```python
from build123d import *

# Parameters (mm, degrees)
SKETCH1_R           = 1
BOSS_EXTRUDE1_DEPTH = 12
SKETCH2_R           = 3.3
CUT_EXTRUDE1_DEPTH  = 4.5
FILLET1_R           = 1
FILLET2_R           = 1


with BuildPart() as part:
    # Sketch1 → Boss-Extrude1 (new body)
    with BuildSketch(Plane.XY):
        with BuildLine():
            Line((-5.308637939, 12.706986515), (-5.308637939, 23.252630458))
            ThreePointArc((-5.308637939, 23.252630458), (-6.101385458, 28.176893504), (-1.247793812, 27.02821456))
            Line((-1.247793812, 27.02821456), (5.613218796, 27.02821456))
            Line((5.613218796, 27.02821456), (12.714242382, 53.529595368))
            ThreePointArc((12.714242382, 53.529595368), (11.748807445, 55.614439687), (11.81766691, 57.910936764))
            ThreePointArc((11.81766691, 57.910936764), (13.042411781, 58.618043545), (13.749518562, 57.393298673))
            ThreePointArc((13.749518562, 57.393298673), (15.870838906, 53.719064059), (19.54507352, 55.840384403))
            ThreePointArc((19.54507352, 55.840384403), (20.769818391, 56.547491184), (21.476925173, 55.322746313))
            ThreePointArc((21.476925173, 55.322746313), (20.38831068, 53.299491772), (18.50979734, 51.976681098))
            Line((18.50979734, 51.976681098), (9.691362061, 19.065832594))
            Line((9.691362061, 19.065832594), (9.691362061, 16.893784379))
            Line((9.691362061, 16.893784379), (23.198320346, -6.500953627))
            Line((23.198320346, -6.500953627), (18.002167924, -9.500953627))
            Line((18.002167924, -9.500953627), (7.947710262, 7.913877886))
            Line((7.947710262, 7.913877886), (-1.883337786, 7.913877886))
            ThreePointArc((-1.883337786, 7.913877886), (-6.49944061, 8.235537199), (-5.308637939, 12.706986515))
        make_face()
        with Locations((-4.058637939, 25.979808487)):
            Circle(SKETCH1_R, mode=Mode.SUBTRACT)
        with Locations((-4.058637939, 9.979808487)):
            Circle(SKETCH1_R, mode=Mode.SUBTRACT)
    extrude(amount=BOSS_EXTRUDE1_DEPTH)

    # Sketch2 → Cut-Extrude1 (cut)
    with BuildSketch(Plane.XY.offset(12)):
        with Locations((-4.058637939, 9.979808487)):
            Circle(SKETCH2_R)
        with BuildLine():
            Line((-1.360308715, 24.080066558), (2.301920689, 29.28177342))
            Line((2.301920689, 29.28177342), (-2.704987918, 28.989398429))
            ThreePointArc((-2.704987918, 28.989398429), (-7.241406986, 25.108039484), (-1.360308715, 24.080066558))
        make_face()
    cut_extrude1 = extrude(amount=-CUT_EXTRUDE1_DEPTH, mode=Mode.SUBTRACT)

    # Mirror1: Cut-Extrude1 across plane
    add(cut_extrude1.mirror(Plane.XY.offset(6)), mode=Mode.SUBTRACT)

    # Fillet1
    fillet1_edges = [part.edges().sort_by_distance(p)[0] for p in [
        (-5.308637939, 22.925712876, 9.75),
        (-5.308637939, 13.033904097, 9.75),
        (0.715316572, 27.02821456, 9.75),
        (-1.485326696, 7.913877886, 9.75),
        (-5.308637939, 22.925712876, 2.25),
        (-5.308637939, 13.033904097, 2.25),
        (0.715316572, 27.02821456, 2.25),
        (-1.485326696, 7.913877886, 2.25),
    ]]
    fillet(fillet1_edges, radius=FILLET1_R)

    # Fillet2
    fillet2_edges = [part.edges().sort_by_distance(p)[0] for p in [
        (23.198320346, -6.500953627, 6),
        (18.002167924, -9.500953627, 6),
    ]]
    fillet(fillet2_edges, radius=FILLET2_R)


solid = part.part
```
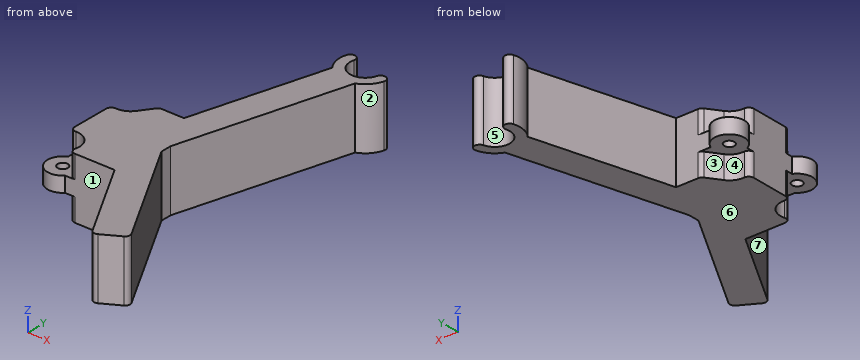
Input: part model. Units: mm. Frame: model coordinates. Face numbers are marked on the shaded views. A direction names the side the tool comes from. Round coordinates to 2 decimals unless told otherwise and drop trailing zeros. Loops run counter-clockwise (first coordinate to the right, second up) from the corner with the lowest first, then second, coordinate; pieces in that order, holes last. Notation, with made-up numbers: (-9, 20.25) - (22, 20.25) arc R14 ccw to (22, 36.25) - close; hole circle Ø7 at (81.5, 36). An arc over 180 degrees is marked (long way). One line per item, written item: value. Start each with the question number.
(1) Section B-B, the plane z = 9. Return loops of the section in (x, y).
(2) Section A-A, the plane x = 16. Return loops of the section in (y, z), plus the area to 3 significant figures.
(3) Ray query, line 1 (Y direction, x = 5, z = 5.75); line 2 (X direction, y = 54, z = 6.25); line 3 (Y direction, x = 20.25, z = 6.5). Return the intervals inside material, ascending. Write a range as [from, to].
(4) Draft query along Y for the marked faces 4, 5, 6 and 7. Return one class per face: +Y half, -Y half, draft (parallel to the pull), parting line (faces both ways), or undercut.
(5) Section C-C, the plane x = 5. Return loops of the section in (y, z).
(6) Section D-D, the plane x = 20.5. Return loops of the section in (y, z), plus the area to 3 significant figures.
(7) Contact query for flat-ended pins moving along their axis: P1, Ø3.5, axis at x = 3.5, z = 4, coming from the +Y side; P2, Ø1.1, axis at y = 18, z = 8.5, coming from the +X side; P3, Ø1, axis at x = 17.5, z = 5.5, coming from the -Y side. Output: stop coordinate, or through.
(8) Access query for the marked faces 1, 2 and 3. Directions: +Z, -Z, +X, -X, +Y, -Y. A direction counts if a zero-diameter tool reaches every point of the face in a straight line with its end or side. Return the directions, or none.
Results below:
1. outline: (-5.31, 14.27) arc R1 ccw to (-4.25, 13.27) arc R3.3 cw to (-0.86, 9.16) arc R1 ccw to (0.11, 7.91) - (7.95, 7.91) - (17.5, -8.63) arc R1 ccw to (18.87, -9) - (22.33, -7) arc R1 ccw to (22.7, -5.63) - (9.69, 16.89) - (9.69, 19.07) - (18.51, 51.98) arc R5 ccw to (21.48, 55.32) arc R1 ccw to (19.55, 55.84) arc R3 cw to (13.75, 57.39) arc R1 ccw to (11.82, 57.91) arc R5 ccw to (12.71, 53.53) - (5.61, 27.03) - (1.23, 27.03) arc R1 ccw to (0.42, 26.6) - (-1.36, 24.08) arc R3.3 cw to (-4.25, 22.69) arc R1 ccw to (-5.31, 21.69) - close
2. outline: (-6.03, 0) - (5.97, 0) - (5.97, 12) - (-6.03, 12) - close; (42.61, 0) - (53.69, 0) - (53.69, 12) - (42.61, 12) - close
2. area: 277 mm^2
3. line 1: [7.91, 27.03]
3. line 2: [12.39, 15.18], [18.11, 20.91]
3. line 3: [-8.2, -1.39], [53.15, 56.55]
4. face 4: +Y half
4. face 5: undercut
4. face 6: draft
4. face 7: -Y half
5. outline: (7.91, 0) - (27.03, 0) - (27.03, 12) - (7.91, 12) - close
6. outline: (-8.06, 0) - (-1.83, 0) - (-1.83, 12) - (-8.06, 12) - close; (53.43, 0) - (56.58, 0) - (56.58, 12) - (53.43, 12) - close
6. area: 113 mm^2
7. P1: y = 27.03
7. P2: x = 9.69
7. P3: y = -9.06
8. face 1: +Z, -Z, -Y
8. face 2: +Z, -Z, +X
8. face 3: -Z, -X, +Y
